from build123d import *

# Parameters (mm, degrees)
F0_R      = 4
F1_DEPTH  = 2
F2_R      = 2.5
F3_DEPTH  = 5
F4_R      = 4
F5_DEPTH  = 2
F6_R      = 2.5
F7_DEPTH  = 24
F8_R      = 4
F9_DEPTH  = 2
F10_R     = 2.5
F11_DEPTH = 16
F12_R     = 4
F13_DEPTH = 2
F14_R     = 2.5
F15_DEPTH = 24
F16_R     = 4
F17_DEPTH = 2
F18_R     = 2.5
F19_DEPTH = 5
F20_R     = 4
F21_DEPTH = 2


with BuildPart() as f1:
    # F0 (on Right) → F1 (new body)
    with BuildSketch(Plane.YZ):
        Circle(F0_R)
    extrude(amount=F1_DEPTH)

    # F2 (on face) → F3 (join)
    with BuildSketch(Plane.YZ.offset(2)):
        Circle(F2_R)
    extrude(amount=F3_DEPTH)

    # F4 (on face) → F5 (join)
    with BuildSketch(Plane.YZ.offset(7)):
        Circle(F4_R)
    extrude(amount=F5_DEPTH)

    # F6 (on face) → F7 (join)
    with BuildSketch(Plane.YZ.offset(9)):
        Circle(F6_R)
    extrude(amount=F7_DEPTH)

    # F8 (on face) → F9 (join)
    with BuildSketch(Plane.YZ.offset(33)):
        Circle(F8_R)
    extrude(amount=F9_DEPTH)

    # F10 (on face) → F11 (join)
    with BuildSketch(Plane.YZ.offset(35)):
        Circle(F10_R)
    extrude(amount=F11_DEPTH)

    # F12 (on face) → F13 (join)
    with BuildSketch(Plane.YZ.offset(51)):
        Circle(F12_R)
    extrude(amount=F13_DEPTH)

    # F14 (on face) → F15 (join)
    with BuildSketch(Plane.YZ.offset(53)):
        Circle(F14_R)
    extrude(amount=F15_DEPTH)

    # F16 (on face) → F17 (join)
    with BuildSketch(Plane.YZ.offset(77)):
        Circle(F16_R)
    extrude(amount=F17_DEPTH)

    # F18 (on face) → F19 (join)
    with BuildSketch(Plane.YZ.offset(79)):
        Circle(F18_R)
    extrude(amount=F19_DEPTH)

    # F20 (on face) → F21 (join)
    with BuildSketch(Plane.YZ.offset(84)):
        Circle(F20_R)
    extrude(amount=F21_DEPTH)


solid = f1.part
Part model, mm, in its own coordinate system. A direction names the side the tool comes from. Give positions to 0.01 mm unless a question says otherwise; leave off trailing zeros. Write each loop counter-clockwise with the first axis right and the second up, starting at its lowest first coordinate (ties: lowest second). Pieces come first, ordered by that corner, then holes.
1) Two-plate mould, pull along X, no slides. Class faces 1 (the face through (20.83, -0.54, -2.44)), 2 (the face through (0, 0, 0)), 3 (the face through (51.986, -0.867, -3.905)): released by +X, released by -X, zero draft, split by the parting line, or undercut.
Resolved:
face 1: undercut
face 2: released by -X
face 3: zero draft
2) Cut at A-A on x = 20.5. Write the cut outline in (y, z).
Resolved:
outline: circle Ø5 at (0, 0)
3) Pin check, flat tips, straight feed: pin 1 (1.5 mm diameter, centred on x = 61.5, z = -1, fed in from +Y); pin 2 (1.5 mm diameter, centred on x = 30.5, y = 1.5, fed in from -Z). Stop position of each tip, or through.
Resolved:
pin 1: stops at y = 2.49
pin 2: stops at z = -2.38
4) Which spindle directions (+Z, -Z, +X, -X, +Y, -Y) get a long thin tool onto all of the face, cutting with end or side? Do faces 4 (the face through (64.83, -0.54, -2.44)), 5 (the face through (7.986, -0.867, -3.905)). Say none if no direction does.
Resolved:
face 4: none
face 5: +X, -X
5) Probe L1, parallel to X at y = -0.5, z = -3; L2, parallel to Z at x = 65, y = 0; L3, parallel to Y at x = 39, z = 0.25. List the from-to ranges inside material, lowest first.
Resolved:
L1: x = 0 to 2, 7 to 9, 33 to 35, 51 to 53, 77 to 79, 84 to 86
L2: z = -2.5 to 2.5
L3: y = -2.49 to 2.49
